For this review, take the finished solid that the model builds, in its own axes (mm). A direction names the side the tool comes from. Coordinates: 2 decimals unless noted, no trailing zeros. Order: outer loops, then holes, each group sorted by start corner. A loop starts at its lowest first (then second) coordinate and runs counter-clockwise, first axis right, second up.
from build123d import *


with BuildPart() as part:
    # Sketch1 → Revolve1 (revolve)
    with BuildSketch(Plane(origin=(0, 0, 0), x_dir=(0, 0, -1), z_dir=(1, 0, 0)), mode=Mode.PRIVATE) as revolve1_sk:
        with BuildLine():
            Line((0, 39.05), (0.5, 38.55))
            Line((0.5, 38.55), (10, 38.55))
            Line((10, 38.55), (10.5, 39.05))
            Line((10.5, 39.05), (10.5, 45.575))
            ThreePointArc((10.5, 45.575), (10.382842712, 45.857842712), (10.1, 45.975))
            Line((10.1, 45.975), (4.556372043, 45.975))
            ThreePointArc((4.556372043, 45.975), (4.312230098, 46.013163593), (4.091381488, 46.124013223))
            Line((4.091381488, 46.124013223), (1.5, 47.975))
            Line((1.5, 47.975), (0.4, 47.975))
            ThreePointArc((0.4, 47.975), (0.117157288, 47.857842712), (0, 47.575))
            Line((0, 47.575), (0, 39.05))
        make_face()
    revolve(revolve1_sk.sketch.rotate(Axis((0, 0, 0), (0, 0, -1)), 90), axis=Axis((0, 0, 0), (0, 0, -1)))


solid = part.part
1. The part is to be moulded in two halves that separate along Y. For faces 1 (the face through (-4, -39, 0)), 2 (the face through (-10.02, 45.14, -3.93)), 3 (the face through (17.79, 34.2, -5.32)), say which applies: +Y half, -Y half, draft (parallel to the pull), parting line (faces both ways), or undercut.
Answer below:
face 1: draft
face 2: parting line
face 3: undercut
2. Clearance check with flat-ended pins moving along their axes: pin 1 Ø5 at (y, z) = (12, -8) entering from +X; pin 2 Ø4 at (x, z) = (25.5, -4) entering from -Y; pin 3 Ø6 at (y, z) = (12, -7.5) entering from +X. State where each tip first meets the part, or that it passes through.
Answer below:
pin 1: stops at x = 44.98
pin 2: stops at y = -40.62
pin 3: stops at x = 45.09
3. Take a section at A-A, the plane y = 0. Give the boundary of the cut face in (x, z) (3 decimals), plus the area to 3 significant figures.
Answer below:
outline: (-47.975, -1.5) - (-46.124, -4.091) arc R0.8 cw to (-45.975, -4.556) - (-45.975, -10.1) arc R0.4 ccw to (-45.575, -10.5) - (-39.05, -10.5) - (-38.55, -10) - (-38.55, -0.5) - (-39.05, 0) - (-47.575, 0) arc R0.4 ccw to (-47.975, -0.4) - close; (38.55, -10) - (39.05, -10.5) - (45.575, -10.5) arc R0.4 ccw to (45.975, -10.1) - (45.975, -4.556) arc R0.8 cw to (46.124, -4.091) - (47.975, -1.5) - (47.975, -0.4) arc R0.4 ccw to (47.575, 0) - (39.05, 0) - (38.55, -0.5) - close
area: 167 mm2
4. To check wall thickness, follow L1, parallel to Y at x = 0, z = -6 (3 decimals); L2, parallel to X at y = -16.5, z = -2.5; L3, parallel to Y at x = 0, z = -2.5. State the ranges of each line that lie inside material, in increasing order.
Answer below:
L1: y = -45.975 to -38.55, 38.55 to 45.975
L2: x = -44.29 to -34.84, 34.84 to 44.29
L3: y = -47.26 to -38.55, 38.55 to 47.26
5. Take a section at C-C, the plane z = -8.75. Give the boundary of the cut face in (x, y) (3 decimals).
Answer below:
outline: circle Ø91.95 at (0, 0); hole circle Ø77.1 at (0, 0)
6. Machinability: for faces 4 (the face through (45.76, -14.41, -0.94)), 5 (the face through (-5.985, -45.584, -7.289)), which of the approach directions +Z, -Z, +X, -X, +Y, -Y give a long, thin tool a straight path to every point of the face, cutting with its end or side? Answer none if there is none.
Answer below:
face 4: +Z, -Z
face 5: -Z
7. Take a section at D-D, the plane z = -3. Give the boundary of the cut face in (x, y), plus the area to 3 significant figures.
Answer below:
outline: circle Ø93.81 at (0, 0); hole circle Ø77.1 at (0, 0)
area: 2,240 mm2
